Geometry: final body of the model. Coordinates: model frame, mm. Round coordinates to 2 decimals unless told otherwise and drop trailing zeros. Loops run counter-clockwise (first coordinate to the right, second up) from the corner with the lowest first, then second, coordinate; pieces in that order, holes last. Notation, with made-up numbers: (25.5, 62) -> (43.5, 62) arc R20 cw to (43.5, 82) -> close; hole circle Ø7 at (32, 78). An arc over 180 degrees is marked (long way). Answer in a Markdown table with one row per item.
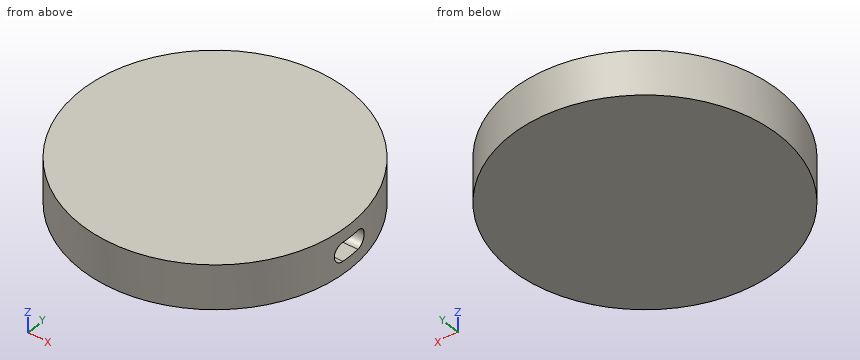
```python
from build123d import *

# Parameters (mm, degrees)
F0_R     = 9.525
F1_DEPTH = 0.79375
F2_R     = 9.525
F2_R_2   = 6.4135
F3_DEPTH = 1.5875
F4_R     = 9.525
F5_DEPTH = 0.79375
F8_DEPTH = 12.7


with BuildPart() as f1:
    # F0 (on Top) → F1 (new body)
    with BuildSketch(Plane.XY):
        Circle(F0_R)
    extrude(amount=F1_DEPTH)

    # F2 (on face) → F3 (join)
    with BuildSketch(Plane.XY.offset(0.79375)):
        Circle(F2_R)
        Circle(F2_R_2, mode=Mode.SUBTRACT)
    extrude(amount=F3_DEPTH)

    # F4 (on face) → F5 (join)
    with BuildSketch(Plane.XY.offset(2.38125)):
        Circle(F4_R)
    extrude(amount=F5_DEPTH)

    # F7 (on offset) → F8 (cut)
    with BuildSketch(Plane.YZ.offset(9.525)):
        with BuildLine():
            Line((0.6731, 2.2606), (-0.6731, 2.2606))
            ThreePointArc((-0.6731, 2.2606), (-1.3462, 1.5875), (-0.6731, 0.9144))
            Line((-0.6731, 0.9144), (0.6731, 0.9144))
            ThreePointArc((0.6731, 0.9144), (1.3462, 1.5875), (0.6731, 2.2606))
        make_face()
    extrude(amount=-F8_DEPTH, mode=Mode.SUBTRACT)


solid = f1.part
```
Item 1: Cut plane C-C (y = -5). Output: boundary loops of the cut face in (x, z) (3 decimals), then the cut area to 3 significant figures.
Answer:
| item | result |
|---|---|
| outline | (-8.107, 0) -> (8.107, 0) -> (8.107, 3.175) -> (-8.107, 3.175) -> close; hole (-4.017, 0.794) -> (4.017, 0.794) -> (4.017, 2.381) -> (-4.017, 2.381) -> close |
| area | 38.7 mm² |
Item 2: Line query: probe 1 along Z at (x, y) = (2.5, 0.25) (3 decimals); probe 2 along Y at (x, z) = (0, 1.3) (1 decimal); probe 3 along Y at (x, z) = (-5, 1.8). Output: solid intervals per line, ascending. Write a range as [from, to].
Answer:
| item | result |
|---|---|
| probe 1 | z = [0, 0.794], [2.381, 3.175] |
| probe 2 | y = [-9.5, -6.4], [6.4, 9.5] |
| probe 3 | y = [-8.11, -4.02], [4.02, 8.11] |
Item 3: Pin query (flat end, axial travel): pin 1 Ø10.5 at (x, y) = (0, 0) entering from -Z; pin 2 Ø1 at (x, z) = (3.5, 2) entering from -Y. Return the tip coordinate at first contact, or that it passes through.
Answer:
| item | result |
|---|---|
| pin 1 | stops at z = 0 |
| pin 2 | stops at y = -9.04 |
Item 4: Cut plane A-A (x = 0). Output: boundary loops of the cut face in (y, z) (1 decimal).
Answer:
| item | result |
|---|---|
| outline | (-9.5, 0) -> (9.5, 0) -> (9.5, 3.2) -> (-9.5, 3.2) -> close; hole (-6.4, 0.8) -> (6.4, 0.8) -> (6.4, 2.4) -> (-6.4, 2.4) -> close |
Item 5: Cut plane D-D (z = 0.3). Output: boundary loops of the cut face in (x, y) (3 decimals), then the cut area to 3 significant figures.
Answer:
| item | result |
|---|---|
| outline | circle Ø19.05 at (0, 0) |
| area | 285 mm² |
